Check sheet for the drawn part. Datum: minimum x, y, z corner. Units: mm. Coordinates: 2 decimals unless noted, no trailing zeros. Order: outer loops, then holes, each group sorted by start corner. A loop starts at its lowest first (then second) coordinate and runs counter-clockwise, first axis right, second up. Notation, with made-up numbers: M 12.5,30.5 L 57.5,30.5 A27 ccw 57.5,55.5 Z; hole C 57.25,-27 d8. An arc over 180 degrees is marked long. Answer in a Markdown table with one row per item. Add a question column.
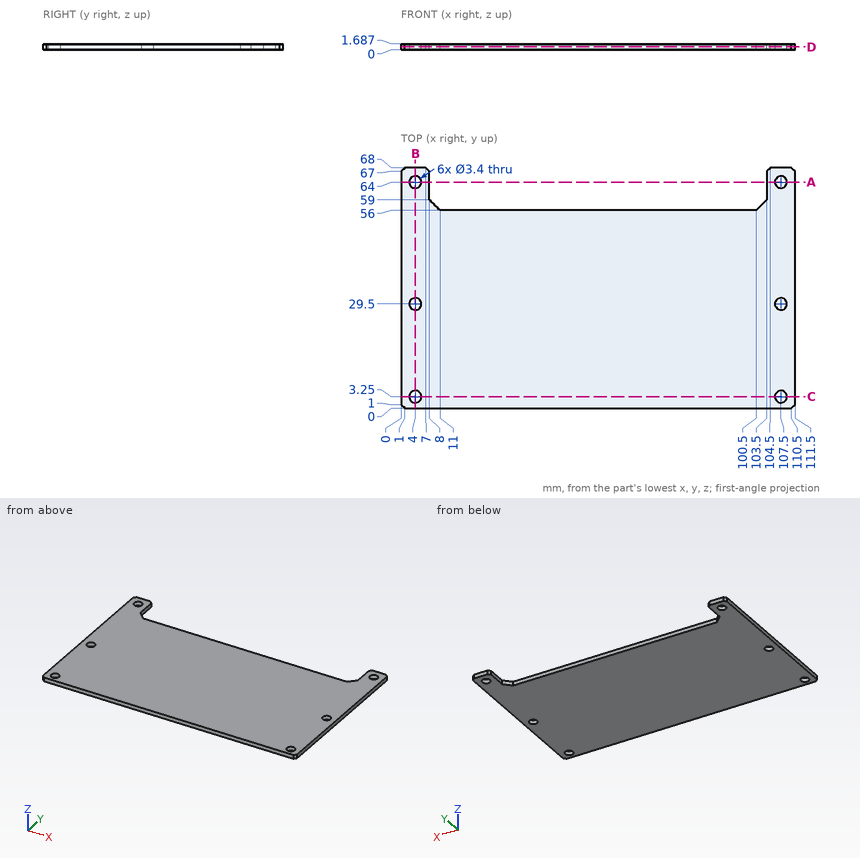
1. Section check C-C on y = 3.25. Enter the section's corners in (x, z).
2. Section check D-D on z = 0.9. Enter the section's corners in (x, y).
3. Go/stop test with flat-tipped pins: pin 1 Ø6 at (x, y) = (24.5, 60.5) entering from -Z; pin 2 Ø0.8 at (x, z) = (75, 1) entering from +Y. Record where each tip stops, or that it passes through.
4. Scan lines: line 1 (Y direction, x = 107.5, z = 0.55); line 2 (X direction, y = 64, z = 1.1); line 3 (X direction, y = 60, z = 0.7). Record each from-to range of solid material in increasing order.
5. Section check B-B on x = 4. Enter the section's corners in (y, z).
6. Section check A-A on y = 64. Enter the section's corners in (x, z).
Result sheet:
| question | item | result |
|---|---|---|
| 1 | outline | M 0,0 L 2.3,0 L 2.3,1.69 L 0,1.69 Z; M 5.7,0 L 105.8,0 L 105.8,1.69 L 5.7,1.69 Z; M 109.2,0 L 111.5,0 L 111.5,1.69 L 109.2,1.69 Z |
| 2 | outline | M 0,1 L 1,0 L 110.5,0 L 111.5,1 L 111.5,67 L 110.5,68 L 104.5,68 L 103.5,67 L 103.5,59 L 100.5,56 L 11,56 L 8,59 L 8,67 L 7,68 L 1,68 L 0,67 Z; hole C 4,3.25 d3.4; hole C 4,29.5 d3.4; hole C 4,64 d3.4; hole C 107.5,3.25 d3.4; hole C 107.5,29.5 d3.4; hole C 107.5,64 d3.4 |
| 3 | pin 1 | through |
| 3 | pin 2 | y = 56 |
| 4 | line 1 | 0 to 1.55, 4.95 to 27.8, 31.2 to 62.3, 65.7 to 68 |
| 4 | line 2 | 0 to 2.3, 5.7 to 8, 103.5 to 105.8, 109.2 to 111.5 |
| 4 | line 3 | 0 to 8, 103.5 to 111.5 |
| 5 | outline | M 0,0 L 1.55,0 L 1.55,1.69 L 0,1.69 Z; M 4.95,0 L 27.8,0 L 27.8,1.69 L 4.95,1.69 Z; M 31.2,0 L 62.3,0 L 62.3,1.69 L 31.2,1.69 Z; M 65.7,0 L 68,0 L 68,1.69 L 65.7,1.69 Z |
| 6 | outline | M 0,0 L 2.3,0 L 2.3,1.69 L 0,1.69 Z; M 5.7,0 L 8,0 L 8,1.69 L 5.7,1.69 Z; M 103.5,0 L 105.8,0 L 105.8,1.69 L 103.5,1.69 Z; M 109.2,0 L 111.5,0 L 111.5,1.69 L 109.2,1.69 Z |
